Source: CAD feature listing. Evaluate the final solid. Frame: model axes, mm. A direction names the side the tool comes from. Coordinates: 2 decimals unless noted, no trailing zeros. Loops run counter-clockwise (first coordinate to the right, second up) from the corner with the lowest first, then second, coordinate; pieces in that order, holes last.
Item 1: Reachability of faces 1 (the flat face through (-5431, 1456, 67)), 2 (the cylindrical face through (-5438.35, 1455.87, 59.27)), 3 (the flat face through (-5432.22, 1454.789, 69.98)) from +Z, -Z, +X, -X, +Y, -Y: full face, straight path, thin tool, end or side. Return the list, or none.
Item 2: Section query A-A, the plane z = 59. Return the cut outline in (x, y), then the cut area to 3 significant figures.
Item 3: Section query D-D, the plane x = -5438. Return the cut outline in (y, z), then the cut area to 3 significant figures.
Item 4: Section query B-B, the plane z = 5.5. Return the cut outline in (x, y), then the cut area to 3 significant figures.
Item 5: Pull-direction query (Y, two-part tool) for faces 4 (the flat face through (-5441.391, 1454, 38)), 5 (the flat face through (-5432.3, 1452.789, 3)), 6 (the flat face through (-5438, 1457.789, 38)); classes: +Y half, -Y half, draft (parallel to the pull), parting line (faces both ways), or undercut.
Item 6: Line query: probe 1 along Z at (x, y) = (-5439.25, 1454); probe 2 along Y at (x, z) = (-5434.25, 8); probe 3 along Y at (x, z) = (-5438.25, 19). Output: solid intervals per line, ascending.
Item 7: Section query C-C, the plane x = -5430.75. State how many separate pieces and enclosed holes the cut face has, then the cut area to 3 significant figures.
```python
from build123d import *

# Parameters (mm, degrees)
EXTRUDE_1_DEPTH     = 78
SKETCH_2_W          = 8
SKETCH_2_H          = 56
CUT_EXTRUDE_1_DEPTH = 9
SKETCH_3_R          = 2.5
CUT_EXTRUDE_2_DEPTH = 9
HOLE_WIZARD_M5_1_D  = 4.2


with BuildPart() as part:
    # 草图1 → 凸台-拉伸1 (new body)
    with BuildSketch(Plane.XY):
        Polygon((-5441.39073995, 1449.788604117), (-5441.39073995, 1457.788604117), (-5427.39073995, 1457.788604117), (-5427.39073995, 1454.788604117), (-5435.39073995, 1454.788604117), (-5435.39073995, 1452.788604117), (-5427.39073995, 1452.788604117), (-5427.39073995, 1449.788604117), align=None)
    extrude(amount=EXTRUDE_1_DEPTH)

    # 草图2 → 切除-拉伸1 (cut, through all)
    with BuildSketch(Plane(origin=(0, 1457.788604117, 0), x_dir=(1, 0, 0), z_dir=(0, 1, 0))):
        with Locations((-5431.39073995, -39)):
            Rectangle(SKETCH_2_W, SKETCH_2_H)
    extrude(amount=-CUT_EXTRUDE_1_DEPTH, mode=Mode.SUBTRACT)

    # 草图3 → 切除-拉伸2 (cut, through all)
    with BuildSketch(Plane(origin=(0, 1457.788604117, 0), x_dir=(1, 0, 0), z_dir=(0, 1, 0))):
        with Locations((-5431.39073995, -72.5)):
            Circle(SKETCH_3_R)
        with Locations((-5431.39073995, -5.5)):
            Circle(SKETCH_3_R)
    extrude(amount=-CUT_EXTRUDE_2_DEPTH, mode=Mode.SUBTRACT)

    # M5 螺纹孔1 (through all)
    with Locations(Plane.ZY.offset(5441.39073995)):
        with Locations((59, 1453.788604117), (19, 1453.788604117)):
            Hole(HOLE_WIZARD_M5_1_D / 2)


solid = part.part
```
Verdict:
1. face 1: +X, +Y, -Y
1. face 2: +X, -X
1. face 3: +Z, -Z, +X
2. outline: (-5441.39, 1449.79) - (-5435.39, 1449.79) - (-5435.39, 1451.69) - (-5441.39, 1451.69) - close; (-5441.39, 1455.89) - (-5435.39, 1455.89) - (-5435.39, 1457.79) - (-5441.39, 1457.79) - close
2. area: 22.8 mm2
3. outline: (1449.79, 0) - (1457.79, 0) - (1457.79, 78) - (1449.79, 78) - close; hole circle Ø4.2 at (1453.79, 19); hole circle Ø4.2 at (1453.79, 59)
3. area: 596 mm2
4. outline: (-5441.39, 1449.79) - (-5433.89, 1449.79) - (-5433.89, 1452.79) - (-5435.39, 1452.79) - (-5435.39, 1454.79) - (-5433.89, 1454.79) - (-5433.89, 1457.79) - (-5441.39, 1457.79) - close; (-5428.89, 1449.79) - (-5427.39, 1449.79) - (-5427.39, 1452.79) - (-5428.89, 1452.79) - close; (-5428.89, 1454.79) - (-5427.39, 1454.79) - (-5427.39, 1457.79) - (-5428.89, 1457.79) - close
4. area: 66.0 mm2
5. face 4: draft
5. face 5: undercut
5. face 6: +Y half
6. probe 1: z = 0 to 16.91, 21.09 to 56.91, 61.09 to 78
6. probe 2: y = 1449.79 to 1452.79, 1454.79 to 1457.79
6. probe 3: y = 1449.79 to 1451.69, 1455.89 to 1457.79
7. separate pieces: 8
7. enclosed holes: 0
7. area: 74.0 mm2
